The listing builds one solid part. Answer for the finished solid, in the listing's coordinates (mm). Face numbers are marked on the shaded views. A direction names the side the tool comes from. Coordinates: 2 decimals unless noted, no trailing zeros. Order: outer loops, then holes, each group sorted by start corner. A loop starts at its lowest first (then second) coordinate and runs counter-clockwise, first axis right, second up. Notation, with made-up numbers: (77.25, 56) -> (121.25, 56) arc R31 cw to (121.25, 92) -> close; hole circle Ø6 at (48.5, 46.5). An arc over 180 degrees is marked (long way). Return JSON: item names as keys, results as strings.
from build123d import *

# Parameters (mm, degrees)
SKETCH1_W           = 7
SKETCH1_H           = 7
BOSS_EXTRUDE1_DEPTH = 3
CUT_EXTRUDE1_DEPTH  = 7
CUT_EXTRUDE2_DEPTH  = 11
SKETCH4_R           = 1.8
CUT_EXTRUDE3_DEPTH  = 0.8
SKETCH5_W           = 0.769230769
SKETCH5_H           = 0.769230769
CUT_EXTRUDE4_DEPTH  = 0.4


with BuildPart() as part:
    # Sketch1 → Boss-Extrude1 (new body)
    with BuildSketch(Plane(origin=(0, 0, 0), x_dir=(1, 0, 0), z_dir=(0, 1, 0))):
        with Locations((3.5, 3.5)):
            Rectangle(SKETCH1_W, SKETCH1_H)
    extrude(amount=BOSS_EXTRUDE1_DEPTH)

    # Sketch2 → Cut-Extrude1 (cut)
    with BuildSketch(Plane.XY):
        Polygon((0, 0), (0.7, 3), (0, 3), align=None)
        Polygon((7, 0), (6.3, 3), (7, 3), align=None)
    extrude(amount=-CUT_EXTRUDE1_DEPTH, mode=Mode.SUBTRACT)

    # Sketch3 → Cut-Extrude2 (cut)
    with BuildSketch(Plane(origin=(0, 0, 0), x_dir=(0, 0, -1), z_dir=(1, 0, 0))):
        Polygon((0, 0), (0.7, 3), (0, 3), align=None)
        Polygon((7, 3), (6.3, 3), (7, 0), align=None)
    extrude(amount=CUT_EXTRUDE2_DEPTH, mode=Mode.SUBTRACT)

    # Sketch4 → Cut-Extrude3 (cut)
    with BuildSketch(Plane.XZ):
        with Locations(Location((3.5, -3.5, 0), (0, 0, 270))):
            Circle(SKETCH4_R)
    extrude(amount=-CUT_EXTRUDE3_DEPTH, mode=Mode.SUBTRACT)

    # Sketch5 → Cut-Extrude4 (cut)
    with BuildSketch(Plane(origin=(0, 3, 0), x_dir=(1, 0, 0), z_dir=(0, 1, 0))):
        with Locations((3.612093963, 5.019669427)):
            Rectangle(SKETCH5_W, SKETCH5_H)
        with BuildLine():
            Line((3.227478578, 3.250438657), (3.996709347, 3.250438657))
            Line((3.996709347, 3.250438657), (3.996709347, 2.691143785))
            add(Edge.make_bspline(
                [(3.996709347, 2.691143785), (3.996354449, 2.637428404), (3.995684356, 2.536006718), (3.983938379, 2.392937498), (3.967617452, 2.267298215), (3.941653281, 2.157473929), (3.906889784, 2.058293502), (3.857739809, 1.967540051), (3.797294746, 1.880692172), (3.723360469, 1.800377793), (3.638309276, 1.726095057), (3.541155635, 1.661498191), (3.434205152, 1.603945573), (3.357369532, 1.573646535), (3.31802345, 1.558130965)],
                knots=[0, 0, 0, 0, 1.347156832, 2.543608823, 3.599300285, 4.522475688, 5.370350604, 6.227678973, 7.103274953, 8.018757603, 8.959280198, 9.929437417, 10.939703653, 12, 12, 12, 12], degree=3))
            Line((3.31802345, 1.558130965), (3.176196527, 1.865823273))
            add(Edge.make_bspline(
                [(3.176196527, 1.865823273), (3.210545046, 1.879869864), (3.276215945, 1.906725527), (3.363744761, 1.959605892), (3.435078145, 2.021405192), (3.491618449, 2.092103782), (3.532319251, 2.173879945), (3.563358678, 2.265654966), (3.580969568, 2.369726497), (3.584571264, 2.442951924), (3.586452937, 2.481207888)],
                knots=[0, 0, 0, 0, 1.115416734, 2.132564161, 3.06091458, 3.941973359, 4.836922823, 5.794989041, 6.848011894, 8, 8, 8, 8], degree=3))
            Line((3.586452937, 2.481207888), (3.227478578, 2.481207888))
            Line((3.227478578, 2.481207888), (3.227478578, 3.250438657))
        make_face()
    extrude(amount=-CUT_EXTRUDE4_DEPTH, mode=Mode.SUBTRACT)


solid = part.part
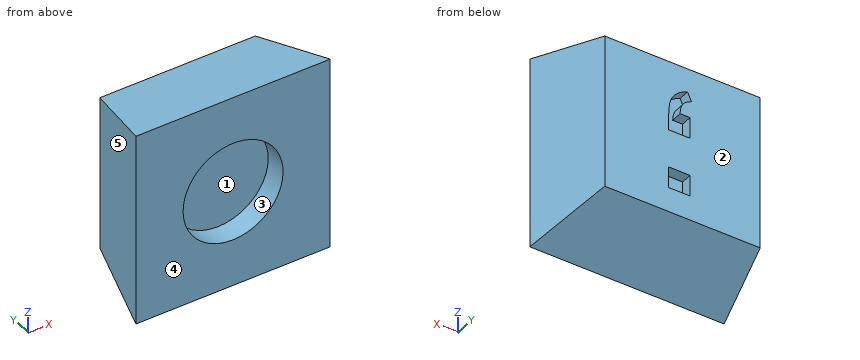
1. Consider line 1 (X direction, y = 0.25, z = -2.5); line 2 (X direction, y = 0.45, z = -3.25) (3 decimals); line 3 (Y direction, x = 3.5, z = -4.25). Determine where each line is inside the solid, lowest interval first. Write a range as from..to.
Answer block:
{"line 1": "x = 0.06..2, 5..6.94", "line 2": "x = 0.105..1.717, 5.283..6.895", "line 3": "y = 0.8..3"}
2. The part is cut by section D-D on y = 1.3. Give the vertices of the cut face in (x, z).
Answer block:
{"outline": "(0.3, -6.7) -> (6.7, -6.7) -> (6.7, -0.3) -> (0.3, -0.3) -> close"}
3. Determine the mould class of the marked faces 3, 4 and 5 for opening direction X: pulls with the +X half, pulls with the -X half, needs draft (parallel to the pull), parting line crosses it, or undercut.
Answer block:
{"face 3": "undercut", "face 4": "needs draft", "face 5": "pulls with the -X half"}
4. For the marked faces 1 and 2, determine the directions among +Z, -Z, +X, -X, +Y, -Y from which every point of the face is accessible in a straight line to the end or side of a thin tool.
Answer block:
{"face 1": "-Y", "face 2": "+Z, -Z, +X, -X, +Y"}
5. The part is cut by section C-C on x = 2. Give the vertices of the cut face in (y, z).
Answer block:
{"outline": "(0, -7) -> (3, -6.3) -> (3, -0.7) -> (0, 0) -> (0, -2.51) -> (0.8, -2.51) -> (0.8, -4.49) -> (0, -4.49) -> close"}
6. The part is cut by section B-B on z = -3.5. Give the vertices of the cut face in (x, y), and give its area (3 significant figures).
Answer block:
{"outline": "(0, 0) -> (1.7, 0) -> (1.7, 0.8) -> (5.3, 0.8) -> (5.3, 0) -> (7, 0) -> (6.3, 3) -> (0.7, 3) -> close", "area": "16.0 mm2"}
7. The part is cut by section A-A on y = 0.35. Give the vertices of the cut face in (x, z).
Answer block:
{"outline": "(0.08, -6.92) -> (6.92, -6.92) -> (6.92, -0.08) -> (0.08, -0.08) -> close; hole circle Ø3.6 at (3.5, -3.5)"}
8. Each of these flat-tipped pins is pushed along its axis until it touches: pin 1 Ø1 at (y, z) = (1, -6) entering from -X; pin 2 Ø1 at (x, y) = (4, 2) entering from +Z; pin 3 Ø1.8 at (x, z) = (3, -3) entering from -Y. Where does it stop, or does it pass through?
Answer block:
{"pin 1": "stops at x = 0.12", "pin 2": "stops at z = -0.35", "pin 3": "stops at y = 0.8"}
